Can you work these out from the drawing? Everything is in mm from the part's minimum corner. A direction names the side the tool comes from. Round coordinates to 2 decimals unless told otherwise and drop trailing zeros. Write each loop counter-clockwise with the first axis right and the second up, starting at its lowest first coordinate (ties: lowest second). Pieces come first, ordered by that corner, then holes.
Q1. If we section it at B-B (y = 123): Please give me the cut outline in (x, z), plus the area to 3 significant figures.
Q2. We'd pull the mould along Y, two halves only. Please class the marked faces 3, 4, 5 and 6: +Y half, -Y half, draft (parallel to the pull), parting line (faces both ways), or undercut.
Q3. For the marked faces 1 and 2, which set-ups out of +Z, -Z, +X, -X, +Y, -Y let a thin tool reach every point of the face, with its end or its side?
Q4. If we section it at A-A (z = 9.5): Please give me the cut outline in (x, y).
Q5. Please list where these lines run through material, in increasing order: line 1 along Y through (x, z) = (83, 64); line 2 along X through (y, z) = (43, 48); line 3 along Z through (x, y) = (12, 107.5).
Q6. If we section it at C-C (x = 47.5): Please give me the cut outline in (y, z), plus the area to 4 significant figures.
Q7. I'm going to push a flat-ended pin straight in: pin 1 Ø12 at (x, y) = (21, 33.5) entering from +Z. Where does the tip first touch, or does it pass through?
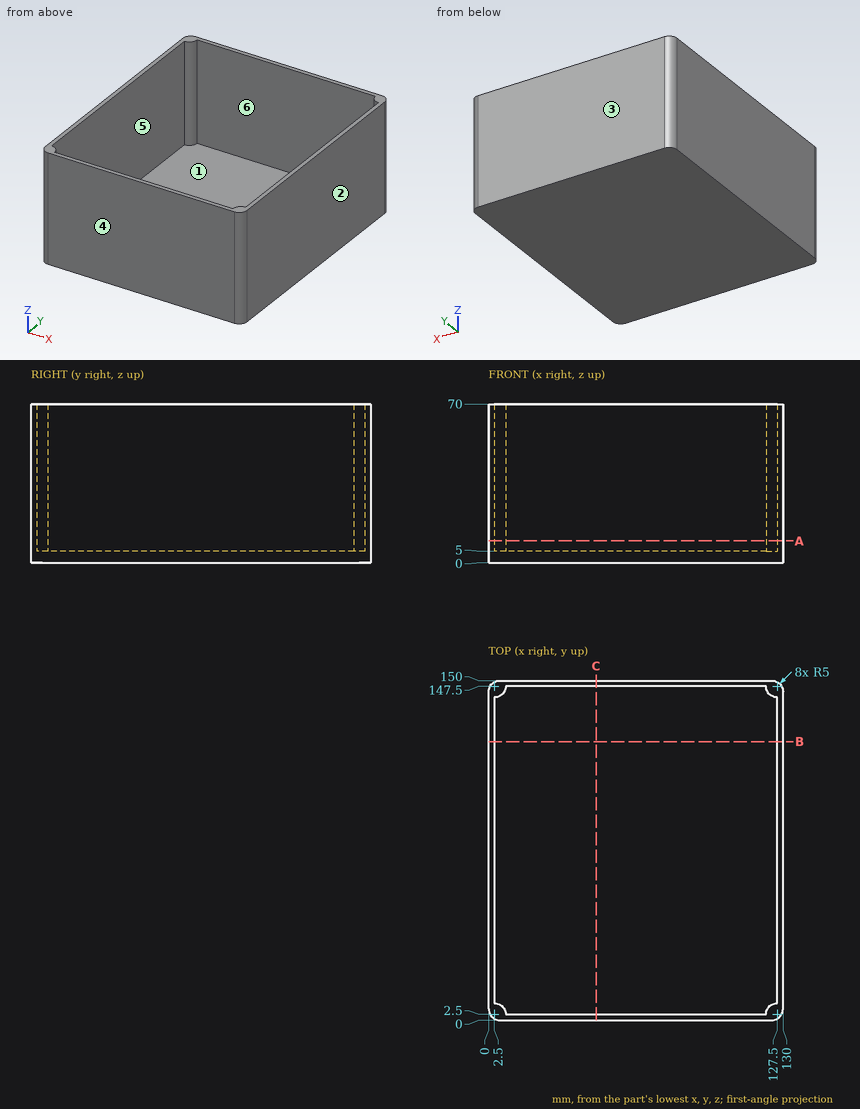
A:
1. outline: (0, 0) - (130, 0) - (130, 70) - (127.5, 70) - (127.5, 5) - (2.5, 5) - (2.5, 70) - (0, 70) - close
1. area: 975 mm2
2. face 3: +Y half
2. face 4: -Y half
2. face 5: undercut
2. face 6: undercut
3. face 1: +Z
3. face 2: +Z, -Z, +X, +Y, -Y
4. outline: (0, 5) arc R5 ccw to (5, 0) - (125, 0) arc R5 ccw to (130, 5) - (130, 145) arc R5 ccw to (125, 150) - (5, 150) arc R5 ccw to (0, 145) - close; hole (2.5, 7.5) arc R5 cw to (7.5, 2.5) - (122.5, 2.5) arc R5 cw to (127.5, 7.5) - (127.5, 142.5) arc R5 cw to (122.5, 147.5) - (7.5, 147.5) arc R5 cw to (2.5, 142.5) - close
5. line 1: y = 0 to 2.5, 147.5 to 150
5. line 2: x = 0 to 2.5, 127.5 to 130
5. line 3: z = 0 to 5
6. outline: (0, 0) - (150, 0) - (150, 70) - (147.5, 70) - (147.5, 5) - (2.5, 5) - (2.5, 70) - (0, 70) - close
6. area: 1,075 mm2
7. pin 1: stops at z = 5
